Part model, mm, in its own coordinate system. A direction names the side the tool comes from. Give positions to 0.01 mm unless a question says otherwise; leave off trailing zeros. Write each loop counter-clockwise with the first axis right and the second up, starting at its lowest first coordinate (ties: lowest second). Pieces come first, ordered by that corner, then holes. Notation, with made-up numbers: (-28, 4) - (-6, 4) arc R32 cw to (-6, 41) - close; hole circle Ø7 at (13, -13.75). An arc over 180 degrees is marked (long way). Answer in a Markdown table with one row per item. Add a question column.
1. Band-saw the part on B-B on x = 1.5. Write the cut outline in (y, z).
2. Probe line 1 along Z through (x, y) = (-5, 2.1); line 2 along X through (y, z) = (1.6, -19); line 3 along Z through (x, y) = (3.5, 2.8). List the from-to ranges inside material, lowest first.
3. Band-saw the part on C-C on x = 5. Write the cut outline in (y, z), plus the area to 3 significant figures.
4. Drop a flat-ended pin along its axis: pin 1 Ø3 at (x, z) = (-5, -24.5) entering from +Y. Give the stop position or say it passes through.
5. Band-saw the part on D-D on y = 2.15. Write the cut outline in (x, z).
6. Which spindle directions (+Z, -Z, +X, -X, +Y, -Y) get a long thin tool onto all of the face, cutting with end or side? Do faces 4 (the cylindrical face through (10.224, 1.479, -20.251)), 5 (the cylindrical face through (-14.797, 1.521, -26.859)). Say none if no direction does.
7. Pull direction Z, two halves, no side cores. Call faces 1 (the cylindrical face through (-3.4, 1.5, 25.7)), 2 (the flat face through (16, 1, 0)), 3 (the flat face through (0, 1, 28)): released by +Z, released by -Z, zero draft, split by the parting line, or undercut.
8. Band-saw the part on A-A on z = 13.5. Write the cut outline in (x, y), plus the area to 3 significant figures.
Autodesk Inventor part; units mm, degrees
ref_plane "YZ Plane" through (0, 0, 0) normal (1, 0, 0) x (0, 1, 0)
ref_plane "XZ Plane" through (0, 0, 0) normal (0, 1, 0) x (-1, 0, 0)
ref_plane "XY Plane" through (0, 0, 0) normal (0, 0, 1) x (1, 0, 0)
sketch "Sketch1" plane through (0, 0, 0) normal (0, 1, 0) x (-1, 0, 0)
  line L0 (9, 20.5) -> (-9, 20.5) construction
  line L1 (-10.5, 19) -> (-10.5, -19) construction
  line L2 (-9, -20.5) -> (9, -20.5) construction
  line L3 (10.5, -19) -> (10.5, 19) construction
  line L4 (10.5, 20.5) -> (-10.5, -20.5) construction
  line L5 (-10.5, 20.5) -> (10.5, -20.5) construction
  circle A0 centre (-5, 24.5) radius 2
  line L6 (0, 0) -> (10.5, 0) construction
  line L7 (0, 0) -> (0, -20.5) construction
  circle A1 centre (5, 24.5) radius 2
  circle A2 centre (-5, -24.5) radius 2
  circle A3 centre (5, -24.5) radius 2
  arc A4 (9, -20.5) -> (10.5, -19) centre (9, -19) ccw
  arc A5 (-10.5, -19) -> (-9, -20.5) centre (-9, -19) ccw construction
  arc A6 (10.5, 19) -> (9, 20.5) centre (9, 19) ccw
  arc A7 (-9, 20.5) -> (-10.5, 19) centre (-9, 19) ccw construction
  line L8 (9, -20.75) -> (-9, -20.75)
  arc A8 (-10.75, -19) -> (-9, -20.75) centre (-9, -19) ccw
  line L9 (-10.75, -19) -> (-10.75, 19)
  arc A9 (-9, 20.75) -> (-10.75, 19) centre (-9, 19) ccw
  line L10 (-9, 20.75) -> (9, 20.75)
  arc A10 (10.75, 19) -> (9, 20.75) centre (9, 19) ccw
  line L11 (10.75, 19) -> (10.75, -19)
  arc A11 (9, -20.75) -> (10.75, -19) centre (9, -19) ccw
  line L12 (16, -28) -> (-16, -28)
  line L13 (-16, -28) -> (-16, 28)
  line L14 (-16, 28) -> (16, 28)
  line L15 (16, 28) -> (16, -28)
  line L16 (16, -28) -> (-16, 28) construction
  line L17 (-16, -28) -> (16, 28) construction
  line L18 (-12.5, -12) -> (-12.5, 12) construction
  point P0 (-12.5, 0)
  dimension "d0" = 21
  dimension "d1" = 41
  dimension "d2" = 4
  dimension "d3" = 5
  dimension "d4" = 24.5
  dimension "d5" = 1.5
  dimension "d6" = 0.25
  dimension "d7" = 32
  dimension "d8" = 56
  dimension "d12" = 24
  dimension "d13" = 3.5
  dimension "d16" = 0
extrude "Extrusion1" add sketch "Sketch1" along normal blind 3
fillet "Fillet1" radius 4 4 edges at (16, 1.5, 28) (-16, 1.5, 28) (16, 1.5, -28) (-16, 1.5, -28)
properties part number "ClawServoPlate" material "Aluminum 6061"
Values:
| question | item | result |
|---|---|---|
| 1 | outline | (0, -28) - (3, -28) - (3, -20.75) - (0, -20.75) - close; (0, 20.75) - (3, 20.75) - (3, 28) - (0, 28) - close |
| 2 | line 1 | z = -28 to -26.5, -22.5 to -20.75, 20.75 to 22.5, 26.5 to 28 |
| 2 | line 2 | x = -16 to -10.75, 10.75 to 16 |
| 2 | line 3 | z = -28 to -25.82, -23.18 to -20.75, 20.75 to 23.18, 25.82 to 28 |
| 3 | outline | (0, -28) - (3, -28) - (3, -26.5) - (0, -26.5) - close; (0, -22.5) - (3, -22.5) - (3, -20.75) - (0, -20.75) - close; (0, 20.75) - (3, 20.75) - (3, 22.5) - (0, 22.5) - close; (0, 26.5) - (3, 26.5) - (3, 28) - (0, 28) - close |
| 3 | area | 19.5 mm² |
| 4 | pin 1 | passes through |
| 5 | outline | (-16, -24) arc R4 ccw to (-12, -28) - (12, -28) arc R4 ccw to (16, -24) - (16, 24) arc R4 ccw to (12, 28) - (-12, 28) arc R4 ccw to (-16, 24) - close; hole (-10.75, -19) arc R1.75 ccw to (-9, -20.75) - (9, -20.75) arc R1.75 ccw to (10.75, -19) - (10.75, 19) arc R1.75 ccw to (9, 20.75) - (-9, 20.75) arc R1.75 ccw to (-10.75, 19) - close; hole circle Ø4 at (-5, -24.5); hole circle Ø4 at (-5, 24.5); hole circle Ø4 at (5, -24.5); hole circle Ø4 at (5, 24.5) |
| 6 | face 4 | +Y, -Y |
| 6 | face 5 | -Z, -X, +Y, -Y |
| 7 | face 1 | undercut |
| 7 | face 2 | zero draft |
| 7 | face 3 | released by +Z |
| 8 | outline | (-16, 0) - (-10.75, 0) - (-10.75, 3) - (-16, 3) - close; (10.75, 0) - (16, 0) - (16, 3) - (10.75, 3) - close |
| 8 | area | 31.5 mm² |
